Autodesk Inventor part; units mm, degrees
ref_plane "YZ Plane" through (0, 0, 0) normal (1, 0, 0) x (0, 1, 0)
ref_plane "XZ Plane" through (0, 0, 0) normal (0, 1, 0) x (-1, 0, 0)
ref_plane "XY Plane" through (0, 0, 0) normal (0, 0, 1) x (1, 0, 0)
sketch "草圖1" plane through (0, 0, 0) normal (0, 1, 0) x (-1, 0, 0)
  line L0 (-33.5, 27) -> (33.5, 27)
  line L1 (33.5, 27) -> (33.5, -27)
  line L2 (33.5, -27) -> (-33.5, -27)
  line L3 (-33.5, -27) -> (-33.5, 27)
  line L4 (-33.5, 27) -> (33.5, -27) construction
  line L5 (33.5, 27) -> (-33.5, -27) construction
  line L6 (43.5, -4.5) -> (33.5, -4.5)
  line L7 (33.5, -4.5) -> (33.5, 4.5)
  line L8 (33.5, 4.5) -> (43.5, 4.5)
  line L9 (43.5, 4.5) -> (43.5, -4.5)
  line L10 (-33.5, -4.5) -> (-43.5, -4.5)
  line L11 (-43.5, -4.5) -> (-43.5, 4.5)
  line L12 (-43.5, 4.5) -> (-33.5, 4.5)
  line L13 (-33.5, 4.5) -> (-33.5, -4.5)
  point P0 (0, 0)
  point P1 (33.5, 0)
  point P2 (-33.5, 0)
  point P3 (-33.5, 4.5)
  point P4 (-33.5, -4.5)
  dimension "d0" = 67
  dimension "d1" = 54
  dimension "d2" = 9
  dimension "d3" = 10
extrude "擠出1" add sketch "草圖1" along normal blind 300
sketch "草圖2" plane through (-33.5, 0, 27) normal (0, 0, 1) x (1, 0, 0)
  circle A0 centre (33.5, 125) radius 30
  line L0 (0, 0) -> (67, 0)
  line L1 (3.5, 125) -> (63.5, 125)
  line L2 (63.5, 125) -> (63.5, -22.0707)
  line L3 (63.5, -22.0707) -> (3.5, -22.0707)
  line L4 (3.5, -22.0707) -> (3.5, 125)
  point P0 (33.5, 0)
  point P1 (33.5, 0)
  point P2 (63.5, 125)
  dimension "d6" = 125
  dimension "d7" = 60
extrude "擠出2" cut sketch "草圖2" against normal through all
sketch "草圖3" plane through (-33.5, 300, 27) normal (0, 0, 1) x (1, 0, 0)
  line L0 (-40.579, -220) -> (107.579, -220)
  line L1 (107.579, -220) -> (107.579, -300)
  line L2 (107.579, -300) -> (-40.579, -300)
  line L3 (-40.579, -300) -> (-40.579, -220)
  point P0 (33.5, -300)
  point P1 (33.5, -300)
  dimension "d10" = 80
extrude "擠出3" cut sketch "草圖3" against normal through all
sketch "草圖4" plane through (33.5, 300, -27) normal (0, 0, -1) x (-1, 0, 0)
  arc A0 (63.5, -175) -> (3.5, -175) centre (33.5, -175) ccw construction
  circle A1 centre (33.5, -159) radius 30
  line L0 (63.5, -220) -> (3.5, -220)
  line L1 (3.5, -220) -> (3.5, -159)
  line L2 (3.5, -159) -> (63.5, -159)
  line L3 (63.5, -159) -> (63.5, -220)
  point P0 (33.5, -300)
  point P1 (63.5, -220)
  dimension "d13" = 16
  dimension "d14" = 60
sketch "草圖5" plane through (-33.5, 300, 27) normal (0, 0, 1) x (1, 0, 0)
  arc A0 (63.5, -175) -> (3.5, -175) centre (33.5, -175) ccw construction
  circle A1 centre (33.5, -157) radius 30
  line L0 (63.5, -220) -> (3.5, -220)
  line L1 (3.5, -220) -> (3.5, -157)
  line L2 (3.5, -157) -> (63.5, -157)
  line L3 (63.5, -157) -> (63.5, -220)
  point P0 (33.5, -300)
  dimension "d15" = 18
  dimension "d16" = 60
loft "斷面混成1" cut profiles "草圖4", "草圖5"
properties part number "Slider-5"
CAD build for the part. Positions are in the model's coordinates, mm. A direction names the side the tool comes from. Coordinates: 2 decimals unless noted, no trailing zeros. Order: outer loops, then holes, each group sorted by start corner. A loop starts at its lowest first (then second) coordinate and runs counter-clockwise, first axis right, second up. Notation, with made-up numbers: (-16, 38.25) -> (28, 38.25) arc R23 cw to (28, 61.25) -> close; hole circle Ø2 at (40, 16.25). An arc over 180 degrees is marked (long way). Answer in a Markdown table with one row per item.
1) Band-saw the part on B-B (x = 37.5). List the corners of the cut face in (y, z).
Check values:
| item | result |
|---|---|
| outline | (80, -4.5) -> (300, -4.5) -> (300, 4.5) -> (80, 4.5) -> close |
2) Flat gauge pins, fed straight in: P1, Ø18, axis at y = 211, z = 12.5, coming from the -X side; P2, Ø11, axis at y = 239.5, z = -21, coming from the -X side; P3, Ø3, axis at y = 268, z = -19, coming from the +X side; P4, Ø11, axis at x = 39.5, y = 222, coming from the -Z side. Where does each tip first touch, or does it go through?
Check values:
| item | result |
|---|---|
| P1 | x = -43.5 |
| P2 | x = -33.5 |
| P3 | x = 33.5 |
| P4 | z = -4.5 |
3) Mould opens along X. For faces 1 (the face through (-39, 188, -4.5)), 2 (the face through (33.5, 188, -16)), 3 (the face through (-30, 111, 0)) say: pulls with the +X half, pulls with the -X half, needs draft (parallel to the pull), parting line crosses it, or undercut.
Check values:
| item | result |
|---|---|
| face 1 | needs draft |
| face 2 | pulls with the +X half |
| face 3 | undercut |
4) Which spindle directions (+Z, -Z, +X, -X, +Y, -Y) get a long thin tool onto all of the face, cutting with end or side? Do faces 4 (the face through (33.5, 188, 16)), 5 (the face through (30, 112, 0)), 6 (the face through (-33.5, 188, 16)). Say none if no direction does.
Check values:
| item | result |
|---|---|
| face 4 | +Z, +X, +Y, -Y |
| face 5 | +Z, -Z, -Y |
| face 6 | +Z, -X, +Y, -Y |
5) Drill centre lines: line 1 (X direction, y = 103, z = -17.5); line 2 (X direction, y = 225, z = 12); line 3 (Z direction, x = 34, y = 230.5). Where is each one in solid material? Low to high.
Check values:
| item | result |
|---|---|
| line 1 | -33.5 to -30, 30 to 33.5 |
| line 2 | -33.5 to 33.5 |
| line 3 | -4.5 to 4.5 |
6) Band-saw the part on A-A (y = 275). List the corners of the cut face in (x, z), and give its area (3 significant figures).
Check values:
| item | result |
|---|---|
| outline | (-43.5, -4.5) -> (-33.5, -4.5) -> (-33.5, -27) -> (33.5, -27) -> (33.5, -4.5) -> (43.5, -4.5) -> (43.5, 4.5) -> (33.5, 4.5) -> (33.5, 27) -> (-33.5, 27) -> (-33.5, 4.5) -> (-43.5, 4.5) -> close |
| area | 3,800 mm2 |
